Geometry check sheet. Reference: the model listing, model coordinates, mm. A direction names the side the tool comes from. Coordinates: 2 decimals unless noted, no trailing zeros. Write each loop counter-clockwise with the first axis right and the second up, starting at its lowest first coordinate (ties: lowest second). Pieces come first, ordered by that corner, then holes. Notation, with made-up numbers: (-7, 3) -> (51, 3) arc R14 cw to (51, 15) -> close; hole circle Ø11 at (10, -13). An arc over 180 degrees is marked (long way). One line per question, with ' | ' between items.
Autodesk Inventor part; units mm, degrees
ref_plane "YZ Plane" through (0, 0, 0) normal (1, 0, 0) x (0, 1, 0)
ref_plane "XZ Plane" through (0, 0, 0) normal (0, 1, 0) x (-1, 0, 0)
ref_plane "XY Plane" through (0, 0, 0) normal (0, 0, 1) x (1, 0, 0)
sketch "Sketch2" plane through (0, 0, 0) normal (0, 0, 1) x (1, 0, 0)
  line L0 (-12.7, -12.7) -> (12.7, -12.7)
  line L1 (12.7, -12.7) -> (12.7, 12.7)
  line L2 (12.7, 12.7) -> (-12.7, 12.7)
  line L3 (-12.7, 12.7) -> (-12.7, -12.7)
  line L4 (-12.7, -12.7) -> (12.7, 12.7) construction
  line L5 (12.7, -12.7) -> (-12.7, 12.7) construction
  line L6 (-9.525, -9.525) -> (9.525, -9.525)
  line L7 (9.525, -9.525) -> (9.525, 9.525)
  line L8 (9.525, 9.525) -> (-9.525, 9.525)
  line L9 (-9.525, 9.525) -> (-9.525, -9.525)
  line L10 (-9.525, -9.525) -> (9.525, 9.525) construction
  line L11 (9.525, -9.525) -> (-9.525, 9.525) construction
  point P0 (0, 0)
  dimension "d0" = 25.4
  dimension "d1" = 25.4
  dimension "d2" = 3.175
  dimension "d3" = 3.175
extrude "Extrusion1" add sketch "Sketch2" along normal mid plane 346.6084
sketch "Sketch5" plane through (12.7, -12.7, -173.3042) normal (1, 0, 0) x (0, 0, -1)
  line L0 (0, 0) -> (-14.6647, 25.4)
  line L1 (0, 25.4) -> (-346.6084, 25.4)
  line L2 (-346.6084, 0) -> (0, 0)
  line L3 (-14.6647, 25.4) -> (0, 25.4)
  line L4 (0, 0) -> (0, 25.4)
  line L5 (0, 25.4) -> (0, 0)
  point P0 (-173.3042, 12.7)
  point P1 (-557.2214, 25.4)
  point P2 (-601.2155, 0)
  dimension "d10" = 60
extrude "Extrusion3" cut sketch "Sketch5" against normal through all
sketch "Sketch6" plane through (12.7, -12.7, 173.3042) normal (1, 0, 0) x (0, 0, -1)
  line L0 (0, 0) -> (0, 25.4)
  line L1 (0, 0) -> (25.4, 25.4)
  line L2 (331.9437, 25.4) -> (0, 25.4)
  line L3 (0, 0) -> (346.6084, 0)
  line L4 (25.4, 25.4) -> (0, 25.4)
  line L5 (0, 25.4) -> (0, 0)
  point P0 (173.3042, 12.7)
  dimension "d13" = 45
extrude "Extrusion4" cut sketch "Sketch6" against normal through all
properties part number "aluminumBallHandlerBackLeg" material "Aluminum 6061-AHC"
(1) Material ranges on line 1 (Y direction, x = 8.5, z = -31) (3 decimals); line 2 (Z direction, x = 10.25, y = -2.25), recorded low to high.
Answers below:
line 1: y = -12.7 to -9.525, 9.525 to 12.7 | line 2: z = -167.27 to 162.85
(2) Cross-section at A-A (z = -39). Record the cut outline in (x, y) (3 decimals).
Answers below:
outline: (-12.7, -12.7) -> (12.7, -12.7) -> (12.7, 12.7) -> (-12.7, 12.7) -> close; hole (-9.525, -9.525) -> (9.525, -9.525) -> (9.525, 9.525) -> (-9.525, 9.525) -> close
(3) Cross-section at C-C (y = 3.25). Record the cut outline in (x, z) (3 decimals).
Answers below:
outline: (-12.7, -164.095) -> (-9.525, -164.095) -> (-9.525, 157.354) -> (-12.7, 157.354) -> close; (9.525, -164.095) -> (12.7, -164.095) -> (12.7, 157.354) -> (9.525, 157.354) -> close
(4) Tool access check on faces 4 (the face through (0, 12.7, -8)), 5 (the face through (9.525, 0, -3)). Record the directions out of +Z, -Z, +X, -X, +Y, -Y that give a thin tool (end or side, any length) a straight path to the whole face; none if there is none.
Answers below:
face 4: +Z, -Z, +X, -X, +Y | face 5: +Z, -Z
(5) Draft check along X on faces 1 (the face through (-9.525, 0, -3)), 2 (the face through (12.7, 0, -2)), 3 (the face through (-11.111, -0.178, -166.075)). Enter one of: pulls with the +X half, pulls with the -X half, needs draft (parallel to the pull), parting line crosses it, or undercut.
Answers below:
face 1: undercut | face 2: pulls with the +X half | face 3: needs draft
(6) Cross-section at B-B (x = -6). Record the cut outline in (y, z) (1 decimal).
Answers below:
outline: (-12.7, -173.3) -> (-9.5, -171.5) -> (-9.5, 170.1) -> (-12.7, 173.3) -> close; (9.5, -160.5) -> (12.7, -158.6) -> (12.7, 147.9) -> (9.5, 151.1) -> close
(7) Depth check by flat-ended pin: P1, Ø4, axis at x = -10, y = 0, coming from the -Z side; P2, Ø2, axis at x = 10, y = 5.5, coming from the -Z side. Enter the tip coordinate at first touch or a pass-through.
Answers below:
P1: stops at z = -167.13 | P2: stops at z = -163.37
